```python
from build123d import *

# Parameters (mm, degrees)
BOSS_EXTRUDE1_DEPTH  = 99.695
SKETCH3_W            = 19.05
SKETCH3_H            = 17.78
SKETCH3_R            = 1.6002
MOUNTING_PLATE_DEPTH = 2.54
CHAMFER1_SIZE        = 5.08
CHAMFER2_SIZE        = 2.54
CHAMFER3_SIZE        = 7.62
FILLET1_R            = 3.81


with BuildPart() as part:
    # Sketch2 → Boss-Extrude1 (new, symmetric)
    with BuildSketch(Plane(origin=(0, 0, 0), x_dir=(0, 0, -1), z_dir=(1, 0, 0))):
        Polygon((-10.069102448, 0), (-6.35, 0), (0, 6.35), (0, 50.8), (-2.54, 50.8), (-2.54, 7.402102448), (-7.529102448, 2.413), (-10.069102448, 2.413), align=None)
    extrude(amount=BOSS_EXTRUDE1_DEPTH, both=True)

    # Sketch3 → Mounting-Plate (add)
    with BuildSketch(Plane.XY):
        with Locations((-109.22, 16.51)):
            Rectangle(SKETCH3_W, SKETCH3_H)
        with Locations(Location((-114.3, 21.59, 0), (0, 0, 90))):
            Circle(SKETCH3_R, mode=Mode.SUBTRACT)
        with Locations(Location((-105.41, 12.7, 0), (0, 0, 90))):
            Circle(SKETCH3_R, mode=Mode.SUBTRACT)
    mounting_plate = extrude(amount=MOUNTING_PLATE_DEPTH)

    # Mirror1: Mounting-Plate across plane
    add(mounting_plate.mirror(Plane(origin=(0, 0, 0), x_dir=(0, 0, 1), z_dir=(1, 0, 0))))

    # Chamfer1
    chamfer1_edges = [part.edges().sort_by_distance(p)[0] for p in [
        (-118.745, 7.62, 1.27),
        (118.745, 7.62, 1.27),
    ]]
    chamfer(chamfer1_edges, length=CHAMFER1_SIZE)

    # Chamfer2
    chamfer2_edges = [part.edges().sort_by_distance(p)[0] for p in [
        (-118.745, 25.4, 1.27),
        (118.745, 25.4, 1.27),
    ]]
    chamfer(chamfer2_edges, length=CHAMFER2_SIZE)

    # Chamfer3
    chamfer3_edges = [part.edges().sort_by_distance(p)[0] for p in [
        (99.695, 50.8, 1.27),
        (-99.695, 50.8, 1.27),
    ]]
    chamfer(chamfer3_edges, length=CHAMFER3_SIZE)

    # Fillet1
    fillet1_edges = [part.edges().sort_by_distance(p)[0] for p in [
        (0, 7.402102448, 2.54),
    ]]
    fillet(fillet1_edges, radius=FILLET1_R)
    fillet1_2_edges = [part.edges().sort_by_distance(p)[0] for p in [
        (-99.695, 25.4, 1.27),
    ]]
    fillet(fillet1_2_edges, radius=FILLET1_R)
    fillet1_3_edges = [part.edges().sort_by_distance(p)[0] for p in [
        (99.695, 25.4, 1.27),
    ]]
    fillet(fillet1_3_edges, radius=FILLET1_R)
    fillet1_4_edges = [part.edges().sort_by_distance(p)[0] for p in [
        (-99.695, 7.62, 1.395547606),
    ]]
    fillet(fillet1_4_edges, radius=FILLET1_R)
    fillet1_5_edges = [part.edges().sort_by_distance(p)[0] for p in [
        (0, 2.413, 7.529102448),
    ]]
    fillet(fillet1_5_edges, radius=FILLET1_R)
    fillet1_6_edges = [part.edges().sort_by_distance(p)[0] for p in [
        (99.695, 7.62, 1.395547606),
    ]]
    fillet(fillet1_6_edges, radius=FILLET1_R)


solid = part.part
```
The listing builds one solid part. Answer for the finished solid, in the listing's coordinates (mm). A direction names the side the tool comes from. Give positions to 0.01 mm unless a question says otherwise; leave off trailing zeros. Order: outer loops, then holes, each group sorted by start corner. A loop starts at its lowest first (then second) coordinate and runs counter-clockwise, first axis right, second up. Notation, with made-up numbers: (6, 24.5) -> (64, 24.5) arc R17 ccw to (64, 31.5) -> close; hole circle Ø10 at (-7, 31.25). An arc over 180 degrees is marked (long way). Answer as a JSON object with one key per item and string values. Group by question number.
Item 1: Consider L1, parallel to X at y = 21.59, z = 0.9 (3 decimals); L2, parallel to X at y = 21, z = 1 (3 decimals); L3, parallel to Z at x = 28.5, y = 17. Determine where each line is inside the solid, lowest interval first. Write a range as from..to.
Item 2: The part is cut by section B-B on y = 35. Write down the section's boundary in (x, z) (3 decimals).
Item 3: Flat-ended cylindrical pins translate along their axes: pin 1 (3 mm diameter, centred on x = 16.5, y = 39.5, fed in from +Z); pin 2 (1.3 mm diameter, centred on x = 110, z = 1.5, fed in from +Y); pin 3 (1.9 mm diameter, centred on x = 105.41, y = 12.7, fed in from +Z); pin 4 (0.8 mm diameter, centred on y = 36.5, z = 1.5, fed in from -X) (3 decimals). Find the tip coordinate at first contact, or state that the pin passes through.
Item 4: The part is cut by section A-A on x = -43.5. Write down the section's boundary in (y, z).
Item 5: A tool of negligible diameter and unlimited length cuts with its end or side. For faces 1 (the flat face through (95.938, 46.937, 1.252)), 2 (the flat face through (99.695, 2, 7)), 3 (the flat face through (2, 30, 2.54)), 4 (the flat face through (-99.695, 2, 7)), from which of +Z, -Z, +X, -X, +Y, -Y can it reach the whole face along a straight path? Write none if from no direction.
Result set:
{
 "1": {"L1": "-118.745..-115.9, -112.7..112.7, 115.9..118.745", "L2": "-118.745..-115.787, -112.813..112.813, 115.787..118.745", "L3": "0..2.54"},
 "2": {"outline": "(-99.695, 0) -> (99.695, 0) -> (99.695, 2.54) -> (-99.695, 2.54) -> close"},
 "3": {"pin 1": "z = 2.54", "pin 2": "y = 25.4", "pin 3": "through", "pin 4": "x = -99.695"},
 "4": {"outline": "(0, 6.35) -> (6.35, 0) -> (50.8, 0) -> (50.8, 2.54) -> (8.98, 2.54) arc R3.81 cw to (6.29, 3.66) -> (3.53, 6.41) arc R3.81 cw to (2.41, 9.11) -> (2.41, 10.07) -> (0, 10.07) -> close"},
 "5": {"face 1": "+Z, -Z, +X, +Y", "face 2": "+Z, -Z, +X, -Y", "face 3": "+Z, +X, -X, +Y", "face 4": "+Z, -Z, -X, -Y"}
}
